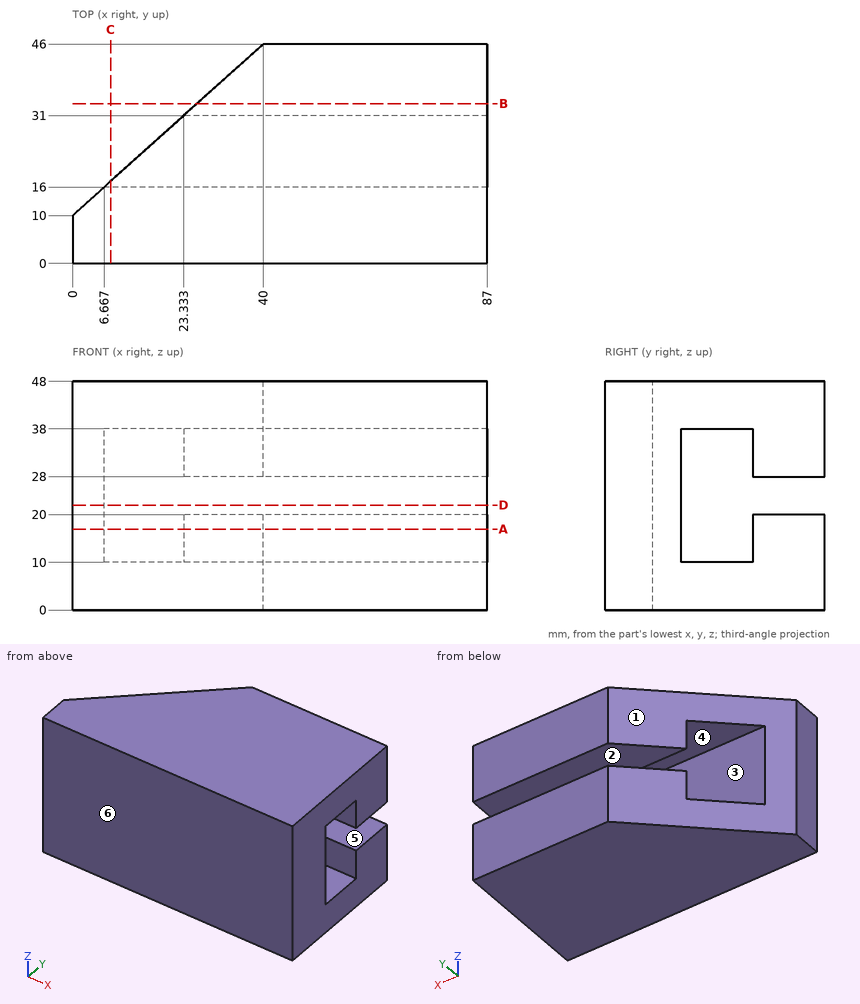
Verification items for this drawing (mm, ordinates from the low corner). A direction names the side the tool comes from. Coordinates: 2 decimals unless noted, no trailing zeros. Order: outer loops, then holes, each group sorted by start corner. A loop starts at its lowest first (then second) coordinate and runs counter-clockwise, first axis right, second up. Notation, with made-up numbers: (37.25, -20.75) - (87.25, -20.75) arc R10 cw to (87.25, -6.75) - close; hole circle Ø10 at (5, 38). An arc over 180 degrees is marked (long way). Use one line per item in the form item = value.
1. Gauge pin test, flat ends, axial feed: pin 1 (1.5 mm diameter, centred on x = 29, z = 43, fed in from +Y) (1 decimal); pin 2 (4 mm diameter, centred on x = 9.5, z = 35.5, fed in from +Y); pin 3 (6 mm diameter, centred on x = 24.5, z = 36, fed in from +Y). Record the tip position at first contact, or that the pin passes through.
Here are the results:
pin_1 = 36.8
pin_2 = 16
pin_3 = 34.75
2. Access from +Z, -Z, +X, -X, +Y, -Y to the whole of each face (thin tool, end or side, straight path). Record for the marked faces 4, 5 and 6.
Here are the results:
face_4 = +X, -X
face_5 = +X, -X, +Y
face_6 = +Z, -Z, +X, -X, -Y
3. Section check C-C (x = 8). Record the boundary of the cut face in (y, z), then the cut area to 3 significant figures.
Here are the results:
outline = (0, 0) - (17.2, 0) - (17.2, 10) - (16, 10) - (16, 38) - (17.2, 38) - (17.2, 48) - (0, 48) - close
area = 792 mm²
4. Draft check along Y on the marked faces 1, 2 and 3. Enter one of: pulls with the +Y half, pulls with the -Y half, needs draft (parallel to the pull), parting line crosses it, or undercut.
Here are the results:
face_1 = pulls with the +Y half
face_2 = needs draft
face_3 = undercut
5. Section check B-B (y = 33.5). Record the boundary of the cut face in (x, z).
Here are the results:
outline = (26.11, 0) - (87, 0) - (87, 20) - (26.11, 20) - close; (26.11, 28) - (87, 28) - (87, 48) - (26.11, 48) - close
6. Scan lines: line 1 (Y direction, x = 78, z = 14.5); line 2 (Z direction, x = 73.5, y = 17); line 3 (Z direction, x = 40.5, y = 32.5). Record each from-to range of solid material in increasing order.
Here are the results:
line_1 = 0 to 16, 31 to 46
line_2 = 0 to 10, 38 to 48
line_3 = 0 to 20, 28 to 48
7. Section check D-D (z = 22). Record the boundary of the cut face in (x, y), then the cut area to 3 significant figures.
Here are the results:
outline = (0, 0) - (87, 0) - (87, 16) - (6.67, 16) - (0, 10) - close
area = 1,370 mm²
8. Section check A-A (z = 17). Record the boundary of the cut face in (x, y), then the cut area to 3 significant figures.
Here are the results:
outline = (0, 0) - (87, 0) - (87, 16) - (6.67, 16) - (0, 10) - close; (23.33, 31) - (87, 31) - (87, 46) - (40, 46) - close
area = 2,200 mm²
